```python
from build123d import *

# Parameters (mm, degrees)
F1_DEPTH       = 135
F2_R           = 1.5
F2_W           = 65
F2_H           = 46
F3_DEPTH       = 3
F4_R           = 2
F5_DEPTH       = 3
F6_SIZE        = 2
F7_R           = 5
F10_DEPTH      = 116
F15_DEPTH      = 64.5
F15_DEPTH_BACK = 64.5
F17_REACH      = 144.7359325659
F19_DEPTH      = 2.9344428022


# Not quite as in the source:
# - a feature names something its author has since deleted; it is built from what else it names


with BuildPart() as f1:
    # F0 (on Right) → F1 (new body)
    with BuildSketch(Plane.YZ):
        with BuildLine():
            Line((-106.670074853, -43.9587721159), (-20, -3))
            Line((-20, -3), (0, -3))
            Line((0, -3), (0, 0))
            Line((0, 0), (-20.6731804218, 0))
            Line((-20.6731804218, 0), (-107.9518930349, -41.2464037506))
            ThreePointArc((-107.9518930349, -41.2464037506), (-115.0819199271, -55.8463352542), (-102.3973475803, -66))
            Line((-102.3973475803, -66), (-20.1261255298, -66))
            Line((-20.1261255298, -66), (-20.1261255298, -56))
            Line((-20.1261255298, -56), (-18.1261255298, -56))
            Line((-18.1261255298, -56), (-18.1261255298, -58.5))
            Line((-18.1261255298, -58.5), (-15.1261255298, -58.5))
            Line((-15.1261255298, -58.5), (-15.1261255298, -53))
            Line((-15.1261255298, -53), (-23.1261255298, -53))
            Line((-23.1261255298, -53), (-23.1261255298, -63))
            Line((-23.1261255298, -63), (-102.3973475803, -63))
            ThreePointArc((-102.3973475803, -63), (-112.154710924, -55.189488657), (-106.670074853, -43.9587721159))
        make_face()
    extrude(amount=F1_DEPTH)

    # F2 (on face) → F3 (cut, through all)
    with BuildSketch(Plane(origin=(0, -3.7741368225, 7.9861945076), x_dir=(1, 0, 0), z_dir=(0, -0.4272727273, 0.9041227884))):
        with Locations((23, -31.0000917132)):
            Circle(F2_R)
        with Locations((111, -31.0000917132)):
            Circle(F2_R)
        with Locations((111, -96.0000917132)):
            Circle(F2_R)
        with Locations((23, -96.0000917132)):
            Circle(F2_R)
        with Locations((67.5, -63.5000917132)):
            Rectangle(F2_W, F2_H)
    extrude(amount=-F3_DEPTH, mode=Mode.SUBTRACT)

    # F4 (on face) → F5 (cut, through all)
    with BuildSketch(Plane.XY):
        with Locations((20, -10.3)):
            Circle(F4_R)
        with Locations((115, -10.3)):
            Circle(F4_R)
    extrude(amount=-F5_DEPTH, mode=Mode.SUBTRACT)

    # F6
    f6_edges = [f1.edges().sort_by_distance(p)[0] for p in [
        (67.5, -15.126126, -58.5),
    ]]
    chamfer(f6_edges, length=F6_SIZE)

    # F7
    f7_edges = [f1.edges().sort_by_distance(p)[0] for p in [
        (67.5, -20, -3),
    ]]
    fillet(f7_edges, radius=F7_R)

    # F9 (on offset) → F10 (cut, through all)
    with BuildSketch(Plane.XY.offset(50)):
        Polygon((26.5695702088, -145.6731804218), (0, -20.6731804218), (0, -145.6731804218), align=None)
        Polygon((135, -145.6731804218), (135, -20.6731804218), (108.4304297912, -145.6731804218), align=None)
    extrude(amount=-F10_DEPTH, mode=Mode.SUBTRACT)

    # F11 (on face) → F12 (join, up to the next surface of F1)
    with BuildSketch(Plane.XY.offset(-63)):
        Polygon((114.6289920234, -102.3973475803), (117.6289920234, -102.3973475803), (134.4786104219, -23.1261255298), (131.4786104219, -23.1261255298), align=None)
    extrude(until=Until.NEXT)

    # F14 (on offset) → F15 (cut, two sides)
    with BuildSketch(Plane.YZ.offset(67.5)) as f15_sk:
        Polygon((-15.1261255298, -53), (-20.1261255298, -53), (-20.1261255298, -56), (-18.1261255298, -56), (-18.1261255298, -58.5), (-17.1261255298, -58.5), (-15.1261255298, -56.5), align=None)
    extrude(amount=-F15_DEPTH, mode=Mode.SUBTRACT)
    extrude(f15_sk.sketch, amount=F15_DEPTH_BACK, mode=Mode.SUBTRACT)

    f17_end = f1.faces().sort_by_distance((10.9056419214, -64.0293542161, -20.4893747382))[0]
    # F16 (on face) → F17 (join, up to a face of the model that its end follows)
    with BuildSketch(Plane.XY.offset(-63)):
        Polygon((0.5213895781, -23.1261255298), (17.3710079766, -102.3973475803), (20.4380297612, -102.3973475803), (3.5884113627, -23.1261255298), align=None)
    f17_long = extrude(amount=F17_REACH, mode=Mode.PRIVATE)
    add(split(f17_long, bisect_by=f17_end, keep=Keep.BOTTOM, mode=Mode.PRIVATE))

    # F18 (on face) → F19 (cut, through all)
    with BuildSketch(Plane(origin=(133.3685883941, -28.3483685838, 0), x_dir=(0.2079116908, 0.9781476007, 0), z_dir=(0.9781476007, -0.2079116908, 0))):
        Polygon((-2.1533435687, -7.9275703375), (-56.6160369654, -33.1032536049), (-56.6160369654, -49.6283268957), (-2.1533435687, -24.4526436284), align=None)
    extrude(amount=-F19_DEPTH, mode=Mode.SUBTRACT)


solid = f1.part
```
Here's how the part is built. I have some questions about the finished solid (model axes, mm). A direction names the side the tool comes from. Coordinates: 2 decimals unless noted, no trailing zeros. Order: outer loops, then holes, each group sorted by start corner. A loop starts at its lowest first (then second) coordinate and runs counter-clockwise, first axis right, second up. Notation, with made-up numbers: (3, 11.25) - (14, 11.25) arc R23 ccw to (14, 27.25) - close; hole circle Ø2 at (61, 28.5). An arc over 180 degrees is marked (long way). One line per question, with ' | ' between items.
(1) Suppose I cut it at D-D on y = -51. List the corners of the cut face in (x, z) for me, and give its area (3 significant figures).
Report:
outline: (6.45, -66) - (128.55, -66) - (128.55, -34.16) - (125.55, -34.45) - (125.55, -63) - (9.51, -63) - (9.51, -17.65) - (35, -17.65) - (35, -14.33) - (6.45, -14.33) - close; (100, -17.65) - (125.55, -17.65) - (125.55, -17.93) - (128.55, -17.64) - (128.55, -14.33) - (100, -14.33) - close | area: 781 mm2
(2) If we mould it in two halves opening along Z, with no side actions, what happens to faces 4 (the flat face through (66.6, -83.1, -29.5)), 5 (the flat face through (3, -18, -55)), 6 (the flat face through (125.044, -53.399, -47.153))? For each: pulls with the +Z half, pulls with the -Z half, needs draft (parallel to the pull), parting line crosses it, or undercut.
Report:
face 4: pulls with the +Z half | face 5: needs draft | face 6: undercut
(3) Suppose I cut it at A-A on y = -10.3. List the corners of the cut face in (x, z) for me, and give its area (3 significant figures).
Report:
outline: (0, -3) - (18, -3) - (18, 0) - (0, 0) - close; (22, -3) - (113, -3) - (113, 0) - (22, 0) - close; (117, -3) - (135, -3) - (135, 0) - (117, 0) - close | area: 381 mm2
(4) Suppose I cut it at B-B on x = 98. List the corners of the cut face in (y, z) for me.
Report:
outline: (-107.95, -41.25) arc R13 ccw to (-102.4, -66) - (-20.13, -66) - (-20.13, -53) - (-23.13, -53) - (-23.13, -63) - (-102.4, -63) arc R10 cw to (-106.67, -43.96) - (-80.7, -31.69) - (-81.98, -28.97) - close; (-40.39, -9.32) - (-39.11, -12.03) - (-21.01, -3.48) arc R5 cw to (-18.88, -3) - (0, -3) - (0, 0) - (-20.67, 0) - close
(5) For faces 1 (the flat face through (133, -15.126, -55)), 2 (the flat face through (10.26, -54.51, -40.65)), 3 (the flat face through (133, -23.126, -29)), which set-ups out of +Z, -Z, +X, -X, +Y, -Y let a thin tool reach every point of the face, with its end or its side?
Report:
face 1: -Z, +X, -X, +Y | face 2: none | face 3: +X, -X, +Y
(6) Suppose I cut it at C-C on z = -21.5. List the corners of the cut face in (x, y) for me, and give its area (3 significant figures).
Report:
outline: (0.52, -23.13) - (9.67, -66.17) - (35, -66.17) - (35, -59.15) - (11.24, -59.15) - (3.59, -23.13) - close; (100, -66.17) - (125.33, -66.17) - (126.82, -59.17) - (123.95, -58.56) - (123.82, -59.15) - (100, -59.15) - close; (130.05, -29.84) - (132.92, -30.45) - (134.48, -23.13) - (131.48, -23.13) - close | area: 499 mm2
(7) If I drill on L1, parallel to X at y = -10, z = -1; L2, parallel to Y at x = 122.5, z = -20; L3, parallel to Z at x = 64, y = -84, over which ranges is the centre line in solid material (lowest first)?
Report:
L1: x = 0 to 18.02, 21.98 to 113.02, 116.98 to 135 | L2: y = -62.99 to -55.97 | L3: z = -66 to -63, -33.25 to -29.93
(8) Will these pins go through, and if not, where does the flat tip stop? pin 1 (24 mm diameter, centred on x = 70.5, y = -49.5, fed in from +Z); pin 2 (1.5 mm diameter, centred on x = 1.5, z = -32, fed in from +Y); pin 3 (1.5 mm diameter, centred on x = 63, y = -83, fed in from +Z).
Report:
pin 1: stops at z = -7.95 | pin 2: stops at y = -23.13 | pin 3: stops at z = -29.1
